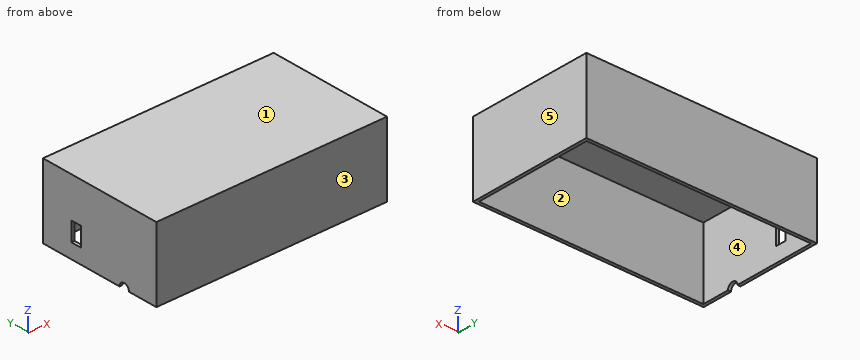
```python
from build123d import *

# Parameters (mm, degrees)
SKIZZE1_W                       = 110
SKIZZE1_H                       = 60
AUFSATZ_LINEAR_AUSTRAGEN1_DEPTH = 35
SCHALE1_T                       = -1.5
SKIZZE3_W                       = 9
SKIZZE3_H                       = 5
SCHNITT_LINEAR_AUSTRAGEN1_DEPTH = 35


with BuildPart() as part:
    # Skizze1 → Aufsatz-Linear austragen1 (new body)
    with BuildSketch(Plane.XY):
        Rectangle(SKIZZE1_W, SKIZZE1_H)
    extrude(amount=AUFSATZ_LINEAR_AUSTRAGEN1_DEPTH)

    # Schale1
    schale1_openings = [part.faces().sort_by_distance(p)[0] for p in [
        (0, 0, 0),
    ]]
    offset(amount=SCHALE1_T, openings=schale1_openings, kind=Kind.INTERSECTION)

    # Skizze3 → Schnitt-Linear austragen1 (cut)
    with BuildSketch(Plane.ZY.offset(55)):
        with BuildLine():
            Line((0, -10.5), (0, -15.5))
            ThreePointArc((0, -15.5), (2.5, -13), (0, -10.5))
        make_face()
        with Locations((11.5, 12.5)):
            Rectangle(SKIZZE3_W, SKIZZE3_H)
    extrude(amount=-SCHNITT_LINEAR_AUSTRAGEN1_DEPTH, mode=Mode.SUBTRACT)


solid = part.part
```
Geometry: final body of the model. Coordinates: model frame, mm. Face numbers are marked on the shaded views. A direction names the side the tool comes from. Coordinates: 2 decimals unless noted, no trailing zeros. Loops run counter-clockwise (first coordinate to the right, second up) from the corner with the lowest first, then second, coordinate; pieces in that order, holes last. Notation, with made-up numbers: (21.5, -15.5) -> (46.5, -15.5) arc R28 ccw to (46.5, 9.5) -> close; hole circle Ø3 at (75, 63.5). An arc over 180 degrees is marked (long way). Use a Markdown table: item, result. Add a question column.
(1) Pin query (flat end, axial travel): pin 1 Ø6 at (x, y) = (-34.5, 7) entering from -Z. Return the tip coordinate at first contact, or that it passes through.
(2) Section query C-C, the plane x = -23. Return loops of the section in (y, z).
(3) Line query: line 1 along X through (y, z) = (-21, 9); line 2 along Y through (x, z) = (22.5, 14); line 3 along Z through (x, y) = (-34, 10). Output: solid intervals per line, ascending.
(4) Access query for the marked faces 1 and 2. Directions: +Z, -Z, +X, -X, +Y, -Y. A direction counts if a zero-diameter tool reaches every point of the face in a straight line with its end or side. Return the directions, or none.
(5) Section query B-B, the plane z = 5.5. Return loops of the section in (x, y).
(6) Section query A-A, the plane y = 12.5. Return loops of the section in (x, z), plus the area to 3 significant figures.
(7) Section query D-D, the plane y = -9. Return loops of the section in (x, z), plus the area to 4 significant figures.
(8) Mould query, pull axis X, two halves, no side actions, for the marked faces 3, 4 and 5. Classes: pulls with the +X half, pulls with the -X half, needs draft (parallel to the pull), parting line crosses it, or undercut.
Answer:
| question | item | result |
|---|---|---|
| 1 | pin 1 | stops at z = 33.5 |
| 2 | outline | (-30, 0) -> (-28.5, 0) -> (-28.5, 33.5) -> (28.5, 33.5) -> (28.5, 0) -> (30, 0) -> (30, 35) -> (-30, 35) -> close |
| 3 | line 1 | x = -55 to -53.5, 53.5 to 55 |
| 3 | line 2 | y = -30 to -28.5, 28.5 to 30 |
| 3 | line 3 | z = 33.5 to 35 |
| 4 | face 1 | +Z, +X, -X, +Y, -Y |
| 4 | face 2 | -Z |
| 5 | outline | (-55, -30) -> (55, -30) -> (55, 30) -> (-55, 30) -> close; hole (-53.5, -28.5) -> (53.5, -28.5) -> (53.5, 28.5) -> (-53.5, 28.5) -> close |
| 6 | outline | (-55, 0) -> (-53.5, 0) -> (-53.5, 7) -> (-55, 7) -> close; (-55, 16) -> (-53.5, 16) -> (-53.5, 33.5) -> (53.5, 33.5) -> (53.5, 0) -> (55, 0) -> (55, 35) -> (-55, 35) -> close |
| 6 | area | 252 mm^2 |
| 7 | outline | (-55, 0) -> (-53.5, 0) -> (-53.5, 33.5) -> (53.5, 33.5) -> (53.5, 0) -> (55, 0) -> (55, 35) -> (-55, 35) -> close |
| 7 | area | 265.5 mm^2 |
| 8 | face 3 | needs draft |
| 8 | face 4 | undercut |
| 8 | face 5 | pulls with the +X half |
